```python
from build123d import *

# Parameters (mm, degrees)
F0_W     = 500
F0_H     = 30
F1_DEPTH = 300
F2_W     = 30
F2_H     = 30.000001
F3_DEPTH = 45
F4_W     = 30
F4_H     = 30
F5_DEPTH = 45


with BuildPart() as f1:
    # F0 (on Front) → F1 (new body)
    with BuildSketch(Plane.XZ):
        Rectangle(F0_W, F0_H)
    extrude(amount=F1_DEPTH)

    # F2 (on Front) → F3 (cut)
    with BuildSketch(Plane.XZ):
        with Locations((65, 0)):
            Rectangle(F2_W, F2_H)
    extrude(amount=F3_DEPTH, mode=Mode.SUBTRACT)

    # F4 (on Front) → F5 (cut)
    with BuildSketch(Plane.XZ):
        with Locations((-165, 0)):
            Rectangle(F4_W, F4_H)
    extrude(amount=F5_DEPTH, mode=Mode.SUBTRACT)


solid = f1.part
```
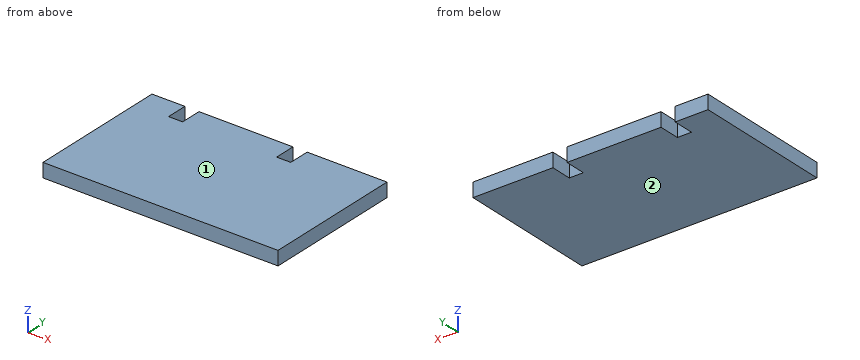
Read the model definition and answer for the solid it produces. Units are mm, in the model's axes. Face numbers are marked on the shaded views. Coordinates: 2 decimals unless noted, no trailing zeros. Loops run counter-clockwise (first coordinate to the right, second up) from the corner with the lowest first, then second, coordinate; pieces in that order, holes last.
(1) Consider line 1 along Y through (x, z) = (-170.5, 10.5). Determine where the line is inside the solid, lowest interval first.
Solution:
line 1: y = -300 to -45
(2) The mould has two halves that part along Z. Classify the marked faces 1 and 2: released by +Z, released by -Z, zero draft, split by the parting line, or undercut.
Solution:
face 1: released by +Z
face 2: released by -Z
(3) The part is cut by section A-A (z = -0.5). Determine the outline of the cut face in (x, y).
Solution:
outline: (-250, -300) - (250, -300) - (250, 0) - (80, 0) - (80, -45) - (50, -45) - (50, 0) - (-150, 0) - (-150, -45) - (-180, -45) - (-180, 0) - (-250, 0) - close
(4) A flat-ended cylindrical pin translates along its axis: pin 1 Ø9 at (x, z) = (-159.5, 4) entering from +Y. Find the tip coordinate at first contact, or state that the pin passes through.
Solution:
pin 1: stops at y = -45
